Part model, mm, in its own coordinate system. Face numbers are marked on the shaded views. A direction names the side the tool comes from. Give positions to 0.01 mm unless a question says otherwise; leave off trailing zeros. Write each loop counter-clockwise with the first axis right and the second up, starting at its lowest first coordinate (ties: lowest second). Pieces come first, ordered by that corner, then holes.
```python
from build123d import *

# Parameters (mm, degrees)
BOSS_EXTRUDE2_DEPTH = 12
SKETCH3_R           = 5
SKETCH3_R_2         = 2.3
CUT_EXTRUDE1_DEPTH  = 13
SKETCH5_R           = 1.25
BOSS_EXTRUDE3_DEPTH = 16
BOSS_EXTRUDE4_DEPTH = 11
CUT_EXTRUDE2_DEPTH  = 3
FILLET1_R           = 0.5
FILLET2_R           = 1
SKETCH9_W           = 5.813805644
SKETCH9_H           = 18.3
SKETCH9_W_2         = 6.1
SKETCH9_H_2         = 7
CUT_EXTRUDE3_DEPTH  = 13
FILLET3_R           = 2


with BuildPart() as part:
    # Sketch1 → Boss-Extrude2 (new body)
    with BuildSketch(Plane(origin=(0, 0, 0), x_dir=(1, 0, 0), z_dir=(0, 1, 0))):
        Polygon((27.85, 13.15), (-18.275666287, 13.15), (-18.813805644, 13.15), (-28.367839887, 0), (-18.813805644, -13.15), (-18.275666287, -13.15), (27.85, -13.15), align=None)
    extrude(amount=-BOSS_EXTRUDE2_DEPTH)

    # Sketch3 → Cut-Extrude1 (cut, through all)
    with BuildSketch(Plane(origin=(0, 0, 0), x_dir=(1, 0, 0), z_dir=(0, 1, 0))):
        Circle(SKETCH3_R)
        with Locations((11.45, 0)):
            Circle(SKETCH3_R_2)
    extrude(amount=-CUT_EXTRUDE1_DEPTH, mode=Mode.SUBTRACT)

    # Sketch5 → Boss-Extrude3 (add)
    with BuildSketch(Plane(origin=(0, 0, 0), x_dir=(1, 0, 0), z_dir=(0, 1, 0))):
        with Locations((20.95, -8.75)):
            Circle(SKETCH5_R)
        with Locations((20.95, 8.75)):
            Circle(SKETCH5_R)
    extrude(amount=BOSS_EXTRUDE3_DEPTH)

    # Sketch6 → Boss-Extrude4 (add)
    with BuildSketch(Plane(origin=(0, 0, 0), x_dir=(1, 0, 0), z_dir=(0, 1, 0))):
        Polygon((-26.423567977, 0), (-23.496516994, -4.028740053), (-18.760449017, -2.489898285), (-18.760449017, 2.489898285), (-23.496516994, 4.028740053), align=None)
    extrude(amount=BOSS_EXTRUDE4_DEPTH)

    # Sketch7 → Cut-Extrude2 (cut)
    with BuildSketch(Plane(origin=(0, 11, 0), x_dir=(1, 0, 0), z_dir=(0, 1, 0))):
        Polygon((-26.423567977, 0), (-23.496516994, -4.028740053), (-18.760449017, -2.489898285), (-18.760449017, 2.489898285), (-23.496516994, 4.028740053), align=None)
        Polygon((-24.940286405, 0), (-23.038157781, -2.618055448), (-19.960449017, -1.618047251), (-19.960449017, 1.618047251), (-23.038157781, 2.618055448), align=None, mode=Mode.SUBTRACT)
    extrude(amount=-CUT_EXTRUDE2_DEPTH, mode=Mode.SUBTRACT)

    # Fillet1
    fillet1_edges = [part.edges().sort_by_distance(p)[0] for p in [
        (-23.496516994, 4, -4.028740053),
        (-18.760449017, 4, -2.489898285),
        (-18.760449017, 4, 2.489898285),
        (-23.496516994, 4, 4.028740053),
        (-26.423567977, 4, 0),
    ]]
    fillet(fillet1_edges, radius=FILLET1_R)

    # Fillet2
    fillet2_edges = [part.edges().sort_by_distance(p)[0] for p in [
        (-18.813805644, -6, -13.15),
        (27.85, -6, -13.15),
        (27.85, -6, 13.15),
        (-18.813805644, -6, 13.15),
        (-28.367839887, -6, 0),
    ]]
    fillet(fillet2_edges, radius=FILLET2_R)

    # Sketch9 → Cut-Extrude3 (cut, through all)
    with BuildSketch(Plane(origin=(0, 0, 0), x_dir=(1, 0, 0), z_dir=(0, 1, 0))):
        with Locations((-11.906902822, 0)):
            Rectangle(SKETCH9_W, SKETCH9_H)
        with Locations((20.8, 0)):
            Rectangle(SKETCH9_W_2, SKETCH9_H_2)
    extrude(amount=-CUT_EXTRUDE3_DEPTH, mode=Mode.SUBTRACT)

    # Fillet3
    fillet3_edges = [part.edges().sort_by_distance(p)[0] for p in [
        (-9, -6, -9.15),
        (-9, -6, 9.15),
        (-14.813805644, -6, 9.15),
        (-14.813805644, -6, -9.15),
        (17.75, -6, 3.5),
        (17.75, -6, -3.5),
        (23.85, -6, -3.5),
        (23.85, -6, 3.5),
    ]]
    fillet(fillet3_edges, radius=FILLET3_R)


solid = part.part
```
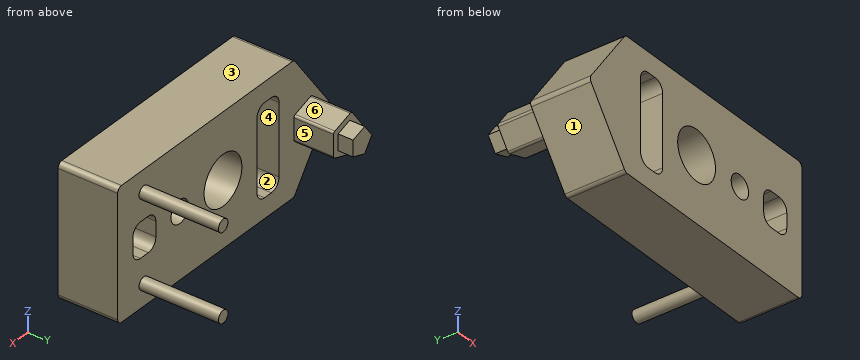
1) Two-plate mould, pull along X, no slides. Class the marked faces 1, 2 and 3: +X half, -X half, draft (parallel to the pull), parting line (faces both ways), or undercut.
Answers follow:
face 1: -X half
face 2: undercut
face 3: draft
2) Saw through at A-A, the plane x = 0. Write the cut outline in (y, z).
Answers follow:
outline: (-12, -13.15) - (0, -13.15) - (0, -5) - (-12, -5) - close; (-12, 5) - (0, 5) - (0, 13.15) - (-12, 13.15) - close
3) Saw through at C-C, the plane y = -9.75. Write the cut outline in (x, z), then the cut area to 3 significant figures.
Answers follow:
outline: (-27.94, -0.59) - (-19.11, -12.74) arc R1 ccw to (-18.3, -13.15) - (26.85, -13.15) arc R1 ccw to (27.85, -12.15) - (27.85, 12.15) arc R1 ccw to (26.85, 13.15) - (-18.3, 13.15) arc R1 ccw to (-19.11, 12.74) - (-27.94, 0.59) arc R1 ccw to start; hole (-14.81, -7.15) arc R2 ccw to (-12.81, -9.15) - (-11, -9.15) arc R2 ccw to (-9, -7.15) - (-9, 7.15) arc R2 ccw to (-11, 9.15) - (-12.81, 9.15) arc R2 ccw to (-14.81, 7.15) - close; hole circle Ø10 at (0, 0); hole circle Ø4.6 at (11.45, 0); hole (17.75, -1.5) arc R2 ccw to (19.75, -3.5) - (21.85, -3.5) arc R2 ccw to (23.85, -1.5) - (23.85, 1.5) arc R2 ccw to (21.85, 3.5) - (19.75, 3.5) arc R2 ccw to (17.75, 1.5) - close
area: 1,110 mm2
4) 3-axis set-ups, long thin cutter, end or side, ignore diameter. For the marked faces 4, 5 and 6: which of +Z, -Z, +X, -X, +Y, -Y reach the whole face in a straight line?
Answers follow:
face 4: +Y, -Y
face 5: +Z, -Z, +X, +Y
face 6: +Z, +X, +Y
5) Saw through at B-B, the plane y = 1.5. Write the cut outline in (x, z).
Answers follow:
outline: (-26.21, -0.29) - (-23.71, -3.73) arc R0.5 ccw to (-23.15, -3.92) - (-19.11, -2.6) arc R0.5 ccw to (-18.76, -2.13) - (-18.76, 2.13) arc R0.5 ccw to (-19.11, 2.6) - (-23.15, 3.92) arc R0.5 ccw to (-23.71, 3.73) - (-26.21, 0.29) arc R0.5 ccw to start; circle Ø2.5 at (20.95, -8.75); circle Ø2.5 at (20.95, 8.75)
6) Wall check: L1, parallel to Z at x = 11.45, y = -6.75; L2, parallel to Z at x = 0, y = -9; L3, parallel to X at y = -9.5, z = 0.5 (3 decimals). Give the ranges that are in metal, low to high.
Answers follow:
L1: z = -13.15 to -2.3, 2.3 to 13.15
L2: z = -13.15 to -5, 5 to 13.15
L3: x = -27.998 to -14.814, -9 to -4.975, 4.975 to 9.205, 13.695 to 17.75, 23.85 to 27.85
7) Saw through at D-D, the plane x = 20.95. Write the cut outline in (y, z).
Answers follow:
outline: (-12, -13.15) - (0, -13.15) - (0, -10) - (16, -10) - (16, -7.5) - (0, -7.5) - (0, -3.5) - (-12, -3.5) - close; (-12, 3.5) - (0, 3.5) - (0, 7.5) - (16, 7.5) - (16, 10) - (0, 10) - (0, 13.15) - (-12, 13.15) - close
8) Pin check, flat tips, straight feed: pin 1 Ø3 at (x, z) = (0, -8.5) entering from +Y; pin 2 Ø1.5 at (x, z) = (-22, -0.5) entering from +Y; pin 3 Ø1.3 at (y, z) = (5.5, -1) entering from +X; pin 4 Ø3.5 at (x, z) = (11.45, 0) entering from -Y. Stop position of each tip, or through.
Answers follow:
pin 1: stops at y = 0
pin 2: stops at y = 11
pin 3: stops at x = -18.76
pin 4: passes through
